Can you work these out from the drawing? Everything is in mm from the part's minimum corner. A direction names the side the tool comes from. Round coordinates to 2 decimals unless told otherwise and drop trailing zeros. Loops run counter-clockwise (first coordinate to the right, second up) from the corner with the lowest first, then second, coordinate; pieces in that order, holes last. Notation, with made-up numbers: (-0.75, -40) - (14.25, -40) arc R21 cw to (14.25, -2) - close; hole circle Ø3 at (20.25, 6). An arc over 180 degrees is marked (long way). Answer as a JSON object with one key per item and string values. Group by question number.
1) I want a section at B-B, the plane x = 95. Please give me the cut outline in (y, z).
2) I want a section at D-D, the plane y = 52. Please give me the cut outline in (x, z).
3) Which directions (+Z, -Z, +X, -X, +Y, -Y) give clear straight access to the entire face, cutting with the end or side of a thin tool? Please do the marked faces 5, 6 and 7.
4) Will these pins go through, and if not, where does the flat tip stop? P1, Ø5, axis at x = 21, y = 44, coming from the -Z side; P2, Ø5, axis at x = 59, z = 6.5, coming from the -Y side; P3, Ø6, axis at x = 91, z = 16.5, coming from the +Y side; P4, Ø5, axis at y = 27, z = 9, coming from the +X side.
5) I want a section at A-A, the plane y = 31. Please give me the cut outline in (x, z).
6) I want a section at C-C, the plane z = 8. Please give me the cut outline in (x, y).
7) If I drill on line 1 along X through (y, z) = (26, 6.75); line 2 along Y through (x, z) = (71.5, 3); line 3 along X through (y, z) = (7, 20), over which ranges is the centre line in solid material (lowest first)? Write a range as [from, to].
8) If we mould it in two halves opening along X, with no side actions, what happens to the marked faces 1, 2, 3 and 4? For each: pulls with the +X half, pulls with the -X half, needs draft (parallel to the pull), parting line crosses it, or undercut.
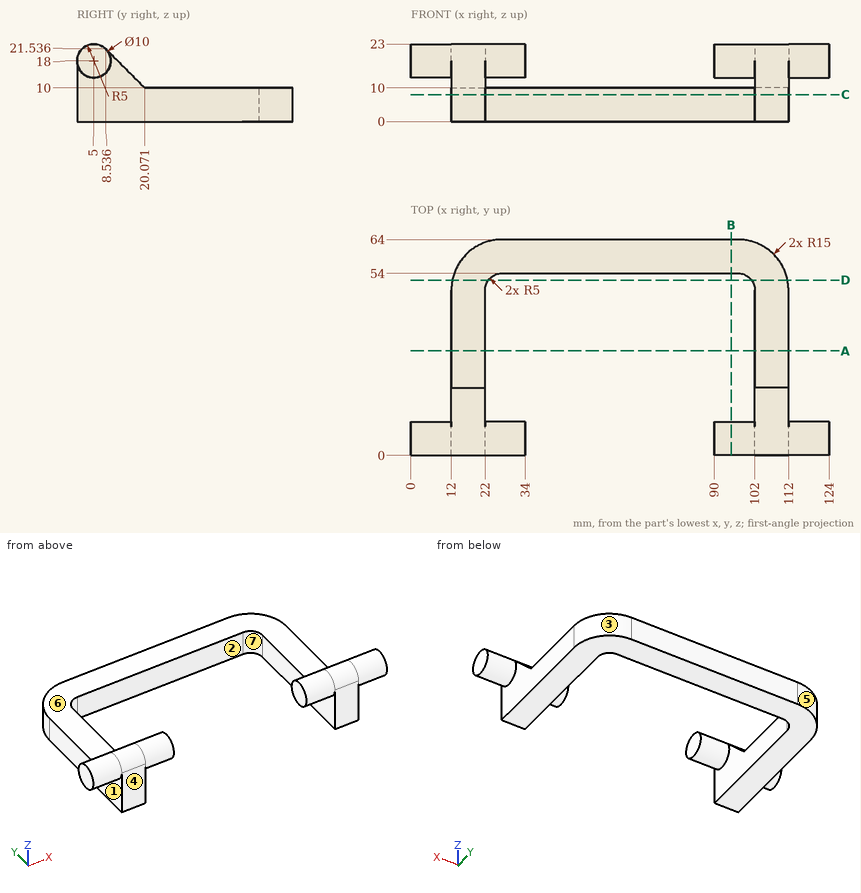
Outcome:
{
 "1": {"outline": "circle Ø10 at (5, 18); (54, 0) - (64, 0) - (64, 10) - (54, 10) - close"},
 "2": {"outline": "(12.3, 0) - (23, 0) - (23, 10) - (12.3, 10) - close; (101, 0) - (111.7, 0) - (111.7, 10) - (101, 10) - close"},
 "3": {"face 5": "+Z, -Z, -X, +Y", "face 6": "+Z, +X, -X, +Y", "face 7": "+Z, -Z, -Y"},
 "4": {"P1": "z = 0", "P2": "y = 54", "P3": "y = 10", "P4": "x = 112"},
 "5": {"outline": "(12, 0) - (22, 0) - (22, 10) - (12, 10) - close; (102, 0) - (112, 0) - (112, 10) - (102, 10) - close"},
 "6": {"outline": "(12, 0) - (22, 0) - (22, 49) arc R5 cw to (27, 54) - (97, 54) arc R5 cw to (102, 49) - (102, 0) - (112, 0) - (112, 49) arc R15 ccw to (97, 64) - (27, 64) arc R15 ccw to (12, 49) - close"},
 "7": {"line 1": "[12, 22], [102, 112]", "line 2": "[54, 64]", "line 3": "[0, 34], [90, 124]"},
 "8": {"face 1": "pulls with the -X half", "face 2": "undercut", "face 3": "pulls with the +X half", "face 4": "needs draft"}
}
